```python
from build123d import *

# Parameters (mm, degrees)
PAD001_DEPTH = 0.55
PAD002_DEPTH = 0.55
PAD_DEPTH    = 4.255
CHAMFER_SIZE = 0.75


with BuildPart() as pad001:
    # Sketch001 → Pad001 (new body, symmetric)
    with BuildSketch(Plane.XZ.offset(2.54)):
        Polygon((-5, 0), (-3.75, 0), (-3.25, 1.35), (3.25, 1.35), (3.75, 0), (5, 0), (5, 0.27), (4, 0.27), (3.5, 1.62), (-3.5, 1.62), (-4, 0.27), (-5, 0.27), align=None)
    extrude(amount=PAD001_DEPTH, both=True)


with BuildPart() as pad002:
    # Sketch002 → Pad002 (new body, symmetric)
    with BuildSketch(Plane.XZ.offset(-2.54)):
        Polygon((-5, 0), (-3.75, 0), (-3.25, 1.35), (3.25, 1.35), (3.75, 0), (5, 0), (5, 0.27), (4, 0.27), (3.5, 1.62), (-3.5, 1.62), (-4, 0.27), (-5, 0.27), align=None)
    extrude(amount=PAD002_DEPTH, both=True)


with BuildPart() as obj1:
    # Sketch → Pad (new body, symmetric)
    with BuildSketch(Plane.XZ):
        Polygon((-3.1, 0.1), (3.1, 0.1), (3.25, 1.35), (3.1, 2.6), (-3.1, 2.6), (-3.25, 1.35), align=None)
    extrude(amount=PAD_DEPTH, both=True)

    # Chamfer
    chamfer_edges = [obj1.edges().sort_by_distance(p)[0] for p in [
        (0, 4.255, 2.6),
    ]]
    chamfer(chamfer_edges, length=CHAMFER_SIZE)

    add(pad001.part)
    add(pad002.part)


solid = obj1.part
```
Work out the finished part from the listing and answer in its coordinate system (mm). A direction names the side the tool comes from. Give positions to 0.01 mm unless a question says otherwise; leave off trailing zeros. Loops run counter-clockwise (first coordinate to the right, second up) from the corner with the lowest first, then second, coordinate; pieces in that order, holes last. Notation, with made-up numbers: (72, 3.5) - (103, 3.5) arc R14 cw to (103, 12.5) - close; hole circle Ø10 at (33, -31). An arc over 180 degrees is marked (long way). Use CSV: the item, a comma, the result in double quotes. Start each with the question number.
(1) Each of these flat-tipped pins is pushed along its axis until it touches: pin 1 (0.5 mm diameter, centred on x = 4.5, y = 2.5, fed in from +Z); pin 2 (0.5 mm diameter, centred on x = 4, z = 0.5, fed in from +Y); pin 3 (0.8 mm diameter, centred on x = 4.5, z = 1, fed in from -Y). Where does it stop, or does it pass through?
(2) Find section B-B, the plane z = 0.55. Determine the outline of the cut face in (x, y) (3 decimals).
(3) Find section D-D, the plane z = 1.1. Determine the outline of the cut face in (x, y) (3 decimals), plus the area to 3 significant figures.
(4) Find section A-A, the plane y = -2.75. Determine the outline of the cut face in (x, z).
(5) Find section C-C, the plane x = -2. Determine the outline of the cut face in (y, z) (3 decimals), plus the area to 3 significant figures.
(6) Determine the mould class of faces 4 (the face through (-3.7, 1.99, 0.6)), 5 (the face through (0, 4.255, 1)), 6 (the face through (0, 0, 2.6)) for opening direction Y: released by +Y, released by -Y, zero draft, split by the parting line, or undercut.
(7) Find the intervals of material crossed by L1, parallel to Z at x = 1.5, y = 1; L2, parallel to X at y = 0.5, z = 0.6; L3, parallel to Y at x = 2.75, z = 2.05 (3 decimals), in increasing order.
(8) A tool of negligible diameter and unlimited length cuts with its end or side. For faces 1 (the face through (-4.4, 2.5, 0)), 2 (the face through (4.5, 2.5, 0.27)), 3 (the face through (-4.5, -2.5, 0.27)), from which of +Z, -Z, +X, -X, +Y, -Y can it reach the whole face along a straight path? Write none if from no direction.
Results found:
1,pin 1,"z = 0.27"
1,pin 2,"y = 3.09"
1,pin 3,"through"
2,outline,"(-3.896, -3.09) - (-3.546, -3.09) - (-3.546, -1.99) - (-3.896, -1.99) - close; (-3.896, 1.99) - (-3.546, 1.99) - (-3.546, 3.09) - (-3.896, 3.09) - close; (-3.154, -4.255) - (3.154, -4.255) - (3.154, 4.255) - (-3.154, 4.255) - close; (3.546, -3.09) - (3.896, -3.09) - (3.896, -1.99) - (3.546, -1.99) - close; (3.546, 1.99) - (3.896, 1.99) - (3.896, 3.09) - (3.546, 3.09) - close"
3,outline,"(-3.693, -3.09) - (-3.343, -3.09) - (-3.343, -1.99) - (-3.693, -1.99) - close; (-3.693, 1.99) - (-3.343, 1.99) - (-3.343, 3.09) - (-3.693, 3.09) - close; (-3.22, -4.255) - (3.22, -4.255) - (3.22, 4.255) - (-3.22, 4.255) - close; (3.343, -3.09) - (3.693, -3.09) - (3.693, -1.99) - (3.343, -1.99) - close; (3.343, 1.99) - (3.693, 1.99) - (3.693, 3.09) - (3.343, 3.09) - close"
3,area,"56.3 mm^2"
4,outline,"(-5, 0) - (-3.75, 0) - (-3.25, 1.35) - (-3.1, 0.1) - (3.1, 0.1) - (3.25, 1.35) - (3.75, 0) - (5, 0) - (5, 0.27) - (4, 0.27) - (3.5, 1.62) - (3.22, 1.62) - (3.1, 2.6) - (-3.1, 2.6) - (-3.22, 1.62) - (-3.5, 1.62) - (-4, 0.27) - (-5, 0.27) - close"
5,outline,"(-4.255, 0.1) - (4.255, 0.1) - (4.255, 1.85) - (3.505, 2.6) - (-4.255, 2.6) - close"
5,area,"21.0 mm^2"
6,face 4,"undercut"
6,face 5,"released by +Y"
6,face 6,"zero draft"
7,L1,"0.1 to 2.6"
7,L2,"-3.16 to 3.16"
7,L3,"-4.255 to 4.055"
8,face 1,"-Z, +X, -X, +Y, -Y"
8,face 2,"+Z, +X, +Y, -Y"
8,face 3,"+Z, -X, +Y, -Y"
